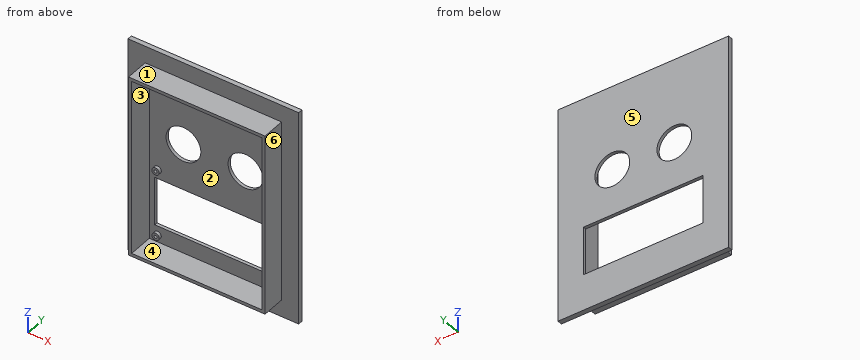
```python
from build123d import *

# Parameters (mm, degrees)
SKETCH1_W           = 139.7
SKETCH1_H           = 177.8
BOSS_EXTRUDE1_DEPTH = 3.81
SKETCH2_W           = 111.76
SKETCH2_H           = 149.86
BOSS_EXTRUDE2_DEPTH = 19.05
SHELL1_START        = -72.39
SHELL1_OUTLINE_W    = 106.68
SHELL1_OUTLINE_H    = 20.32
SHELL1_DEPTH        = 144.78
SKETCH3_R           = 14.25
SKETCH3_W           = 98
SKETCH3_H           = 40
CUT_EXTRUDE1_DEPTH  = 116.346487159
SKETCH4_R           = 3
SKETCH4_R_2         = 1.25
BOSS_EXTRUDE3_DEPTH = 2.54


# Read off the part's stored shape, not the designer's step: Shell1
with BuildPart() as part:
    # Sketch1 → Boss-Extrude1 (new body)
    with BuildSketch(Plane(origin=(0, 0, 0), x_dir=(1, 0, 0), z_dir=(0, 1, 0))):
        Rectangle(SKETCH1_W, SKETCH1_H)
    extrude(amount=BOSS_EXTRUDE1_DEPTH)

    # Sketch2 → Boss-Extrude2 (add)
    with BuildSketch(Plane.XZ):
        Rectangle(SKETCH2_W, SKETCH2_H)
    extrude(amount=BOSS_EXTRUDE2_DEPTH)

    # Shell1 outline → Shell1 (cut)
    with BuildSketch(Plane.XY.offset(SHELL1_START)):
        with Locations((0, -8.89)):
            Rectangle(SHELL1_OUTLINE_W, SHELL1_OUTLINE_H)
    extrude(amount=SHELL1_DEPTH, mode=Mode.SUBTRACT)

    # Sketch3 → Cut-Extrude1 (cut, through all)
    with BuildSketch(Plane(origin=(0, 3.81, 0), x_dir=(1, 0, 0), z_dir=(0, 1, 0))):
        with Locations(Location((-25.4, -19.05, 0), (0, 0, 270))):
            Circle(SKETCH3_R)
        with Locations(Location((25.4, -19.05, 0), (0, 0, 270))):
            Circle(SKETCH3_R)
        with Locations((0, 39.05)):
            Rectangle(SKETCH3_W, SKETCH3_H)
    extrude(amount=-CUT_EXTRUDE1_DEPTH, mode=Mode.SUBTRACT)

    # Sketch4 → Boss-Extrude3 (add)
    # profile 1 of 4: a face of its own
    with BuildSketch(Plane.XZ.offset(-1.27)):
        with Locations(Location((-46.5, -11.55, 0), (0, 0, 90))):
            Circle(SKETCH4_R)
        with Locations(Location((-46.5, -11.55, 0), (0, 0, 270))):
            Circle(SKETCH4_R_2, mode=Mode.SUBTRACT)
    # profile 2 of 4: a face of its own
    with BuildSketch(Plane.XZ.offset(-1.27)):
        with Locations(Location((46.5, -11.55, 0), (0, 0, 90))):
            Circle(SKETCH4_R)
        with Locations(Location((46.5, -11.55, 0), (0, 0, 270))):
            Circle(SKETCH4_R_2, mode=Mode.SUBTRACT)
    # profile 3 of 4: a face of its own
    with BuildSketch(Plane.XZ.offset(-1.27)):
        with Locations(Location((46.5, -66.55, 0), (0, 0, 90))):
            Circle(SKETCH4_R)
        with Locations(Location((46.5, -66.55, 0), (0, 0, 270))):
            Circle(SKETCH4_R_2, mode=Mode.SUBTRACT)
    # profile 4 of 4: a face of its own
    with BuildSketch(Plane.XZ.offset(-1.27)):
        with Locations(Location((-46.5, -66.55, 0), (0, 0, 90))):
            Circle(SKETCH4_R)
        with Locations(Location((-46.5, -66.55, 0), (0, 0, 270))):
            Circle(SKETCH4_R_2, mode=Mode.SUBTRACT)
    extrude(amount=BOSS_EXTRUDE3_DEPTH)


solid = part.part
```
Work out the finished part from the listing and answer in its coordinate system (mm). Face numbers are marked on the shaded views. A direction names the side the tool comes from. Give positions to 0.01 mm unless a question says otherwise; leave off trailing zeros. Write each loop counter-clockwise with the first axis right and the second up, starting at its lowest first coordinate (ties: lowest second). Pieces come first, ordered by that corner, then holes. Notation, with made-up numbers: (70.5, -39.75) -> (113.5, -39.75) arc R19 cw to (113.5, -33.75) -> close; hole circle Ø9 at (16.25, 19). An arc over 180 degrees is marked (long way). Write item = value, one per line.
Q1. Flat-ended cylindrical pins translate along their axes: pin 1 Ø10 at (y, z) = (-6.5, -0.5) entering from +X; pin 2 Ø0.8 at (x, z) = (46.5, -11) entering from -Y; pin 3 Ø1.5 at (y, z) = (-3, 48) entering from -X. Find the tip coordinate at first contact, or state that the pin passes through.
Computed values:
pin_1 = 55.88
pin_2 = 1.27
pin_3 = -55.88
Q2. Section C-C on x = -25.4 is taken. Determine the outline of the cut face in (y, z), and give its area (3 significant figures).
Computed values:
outline = (-19.05, -74.93) -> (0, -74.93) -> (0, -88.9) -> (3.81, -88.9) -> (3.81, -59.05) -> (1.27, -59.05) -> (1.27, -72.39) -> (-19.05, -72.39) -> close; (-19.05, 72.39) -> (1.27, 72.39) -> (1.27, 33.3) -> (3.81, 33.3) -> (3.81, 88.9) -> (0, 88.9) -> (0, 74.93) -> (-19.05, 74.93) -> close; (1.27, -19.05) -> (3.81, -19.05) -> (3.81, 4.8) -> (1.27, 4.8) -> close
area = 416 mm^2
Q3. A tool of negligible diameter and unlimited length cuts with its end or side. For the marked faces 1 and 2, from which of +Z, -Z, +X, -X, +Y, -Y can it reach the whole face along a straight path? Write none if from no direction.
Computed values:
face_1 = +Z, +X, -X, -Y
face_2 = -Y
Q4. Section B-B on y = -9.5 is taken. Determine the outline of the cut face in (x, z).
Computed values:
outline = (-55.88, -74.93) -> (55.88, -74.93) -> (55.88, 74.93) -> (-55.88, 74.93) -> close; hole (-53.34, -72.39) -> (53.34, -72.39) -> (53.34, 72.39) -> (-53.34, 72.39) -> close
Q5. Section D-D on z = -37.5 is taken. Determine the outline of the cut face in (x, y).
Computed values:
outline = (-69.85, 0) -> (-55.88, 0) -> (-55.88, -19.05) -> (-53.34, -19.05) -> (-53.34, 1.27) -> (-49, 1.27) -> (-49, 3.81) -> (-69.85, 3.81) -> close; (49, 1.27) -> (53.34, 1.27) -> (53.34, -19.05) -> (55.88, -19.05) -> (55.88, 0) -> (69.85, 0) -> (69.85, 3.81) -> (49, 3.81) -> close
Q6. Consider line 1 along X through (y, z) = (0.4, -66.55); line 2 along X through (y, z) = (-6.5, 59.5); line 3 along Z through (x, y) = (-39, -10). Determine where each line is inside the solid, lowest interval first.
Computed values:
line_1 = -69.85 to -53.34, -49.5 to -47.75, -45.25 to -43.5, 43.5 to 45.25, 47.75 to 49.5, 53.34 to 69.85
line_2 = -55.88 to -53.34, 53.34 to 55.88
line_3 = -74.93 to -72.39, 72.39 to 74.93
Q7. Section A-A on z = 19.05 is taken. Determine the outline of the cut face in (x, y).
Computed values:
outline = (-69.85, 0) -> (-55.88, 0) -> (-55.88, -19.05) -> (-53.34, -19.05) -> (-53.34, 1.27) -> (-39.65, 1.27) -> (-39.65, 3.81) -> (-69.85, 3.81) -> close; (-11.15, 1.27) -> (11.15, 1.27) -> (11.15, 3.81) -> (-11.15, 3.81) -> close; (39.65, 1.27) -> (53.34, 1.27) -> (53.34, -19.05) -> (55.88, -19.05) -> (55.88, 0) -> (69.85, 0) -> (69.85, 3.81) -> (39.65, 3.81) -> close
Q8. For a pull along X with two mould halves and no side action, classify the marked faces 3, 4, 5 and 6 as pulls with the +X half, pulls with the -X half, needs draft (parallel to the pull), parting line crosses it, or undercut.
Computed values:
face_3 = undercut
face_4 = undercut
face_5 = needs draft
face_6 = pulls with the +X half
